For this review, use the dimensioned drawing (mm, ordinates from the lowest corner) and the shaded views. A direction names the side the tool comes from. Give positions to 0.01 mm unless a question says otherwise; leave off trailing zeros. Loops run counter-clockwise (first coordinate to the right, second up) from the corner with the lowest first, then second, coordinate; pieces in that order, holes last. Notation, with made-up numbers: M 10.25,-15 L 30.25,-15 A13 ccw 30.25,6 Z; hole C 3,33 d6. An arc over 180 degrees is marked long. Use one line per item in the form item = value. Start each with the question number.
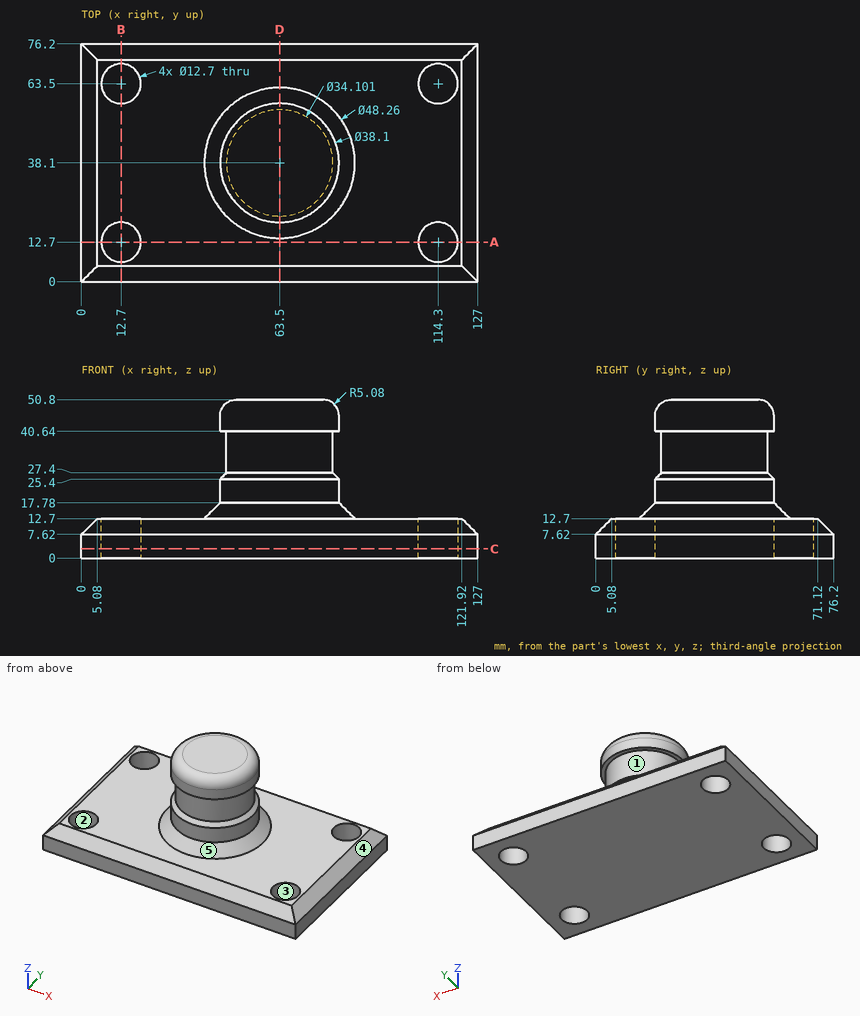
Q1. Take a section at B-B on x = 12.7. Give the boundary of the cut face in (y, z).
Q2. Take a section at C-C on z = 3. Give the boundary of the cut face in (x, y).
Q3. Take a section at A-A on y = 12.7. Give the boundary of the cut face in (x, z).
Q4. For the marked faces 1 and 2, list the 3-axis set-ups (+Z, -Z, +X, -X, +Y, -Y) from which the entire face can be reached by the end or side of a thin tool; tool diameter is ignored.
Q5. The part is to be moulded in two halves that separate along X. For the marked faces 3, 4 and 5, say which applies: pulls with the +X half, pulls with the -X half, needs draft (parallel to the pull), parting line crosses it, or undercut.
Q6. Clearance check with flat-ended pins moving along their axes: pin 1 Ø1.5 at (x, y) = (15.5, 28) entering from -Z; pin 2 Ø20.5 at (x, y) = (12.7, 12.7) entering from +Z; pin 3 Ø6 at (x, z) = (59, 30.5) entering from -Y; pin 4 Ø1.5 at (y, z) = (24.5, 26) entering from -X (1 decimal). State where each tip first meets the part, or that it passes through.
Q7. Wall thickness on probe 1 along Y at (x, z) = (114, 5); probe 2 along X at (y, z) = (63, 5); probe 3 along Y at (x, z) = (12.7, 9): over which ranges is each line inside the solid? List them lowest first.
Q8. Take a section at D-D on x = 63.5. Give the boundary of the cut face in (y, z).
Response values:
q1.outline = M 0,0 L 6.35,0 L 6.35,12.7 L 5.08,12.7 L 0,7.62 Z; M 19.05,0 L 57.15,0 L 57.15,12.7 L 19.05,12.7 Z; M 69.85,0 L 76.2,0 L 76.2,7.62 L 71.12,12.7 L 69.85,12.7 Z
q2.outline = M 0,0 L 127,0 L 127,76.2 L 0,76.2 Z; hole C 12.7,12.7 d12.7; hole C 12.7,63.5 d12.7; hole C 114.3,12.7 d12.7; hole C 114.3,63.5 d12.7
q3.outline = M 0,0 L 6.35,0 L 6.35,12.7 L 5.08,12.7 L 0,7.62 Z; M 19.05,0 L 107.95,0 L 107.95,12.7 L 19.05,12.7 Z; M 120.65,0 L 127,0 L 127,7.62 L 121.92,12.7 L 120.65,12.7 Z
q4.face_1 = none
q4.face_2 = +Z, -Z
q5.face_3 = undercut
q5.face_4 = pulls with the +X half
q5.face_5 = parting line crosses it
q6.pin_1 = 0
q6.pin_2 = 12.7
q6.pin_3 = 21.12
q6.pin_4 = 49.7
q7.probe_1 = 0 to 6.36, 19.04 to 57.16, 69.84 to 76.2
q7.probe_2 = 0 to 6.37, 19.03 to 107.97, 120.63 to 127
q7.probe_3 = 1.38 to 6.35, 19.05 to 57.15, 69.85 to 74.82
q8.outline = M 0,0 L 76.2,0 L 76.2,7.62 L 71.12,12.7 L 62.23,12.7 L 57.15,17.78 L 57.15,25.4 L 55.15,27.4 L 55.15,40.64 L 57.15,40.64 L 57.15,45.72 A5.08 ccw 52.07,50.8 L 24.13,50.8 A5.08 ccw 19.05,45.72 L 19.05,40.64 L 21.05,40.64 L 21.05,27.4 L 19.05,25.4 L 19.05,17.78 L 13.97,12.7 L 5.08,12.7 L 0,7.62 Z
